The model under review builds one solid part; all positions refer to its coordinate system, in mm. Give positions to 0.01 mm unless a question says otherwise; leave off trailing zeros. Loops run counter-clockwise (first coordinate to the right, second up) from the corner with the lowest first, then second, coordinate; pieces in that order, holes last. Notation, with made-up numbers: (-34.75, -13) - (4.25, -13) arc R29 cw to (4.25, 14) - close; hole circle Ø9 at (48, -36.75). An arc over 180 degrees is marked (long way). Answer as a JSON object with one key per item and string values.
from build123d import *

# Parameters (mm, degrees)
SKETCH1_W           = 12.7
SKETCH1_H           = 12.7
SKETCH1_W_2         = 9.525
SKETCH1_H_2         = 9.525
BOSS_EXTRUDE1_DEPTH = 127
CUT_EXTRUDE1_DEPTH  = 13.7
FILLET1_R           = 1.5875


with BuildPart() as part:
    # Sketch1 → Boss-Extrude1 (new body)
    with BuildSketch(Plane.XY):
        with Locations((6.35, 6.35)):
            Rectangle(SKETCH1_W, SKETCH1_H)
        with Locations((6.35, 6.35)):
            Rectangle(SKETCH1_W_2, SKETCH1_H_2, mode=Mode.SUBTRACT)
    extrude(amount=BOSS_EXTRUDE1_DEPTH)

    # Sketch2 → Cut-Extrude1 (cut, through all)
    with BuildSketch(Plane(origin=(0, 12.7, 0), x_dir=(1, 0, 0), z_dir=(0, 1, 0))):
        Polygon((0, -127), (12.7, -127), (12.7, -114.3), align=None)
    extrude(amount=-CUT_EXTRUDE1_DEPTH, mode=Mode.SUBTRACT)

    # Fillet1
    fillet1_edges = [part.edges().sort_by_distance(p)[0] for p in [
        (12.7, 12.7, 57.15),
        (12.7, 0, 57.15),
        (0, 12.7, 63.5),
        (0, 0, 63.5),
    ]]
    fillet(fillet1_edges, radius=FILLET1_R)


solid = part.part
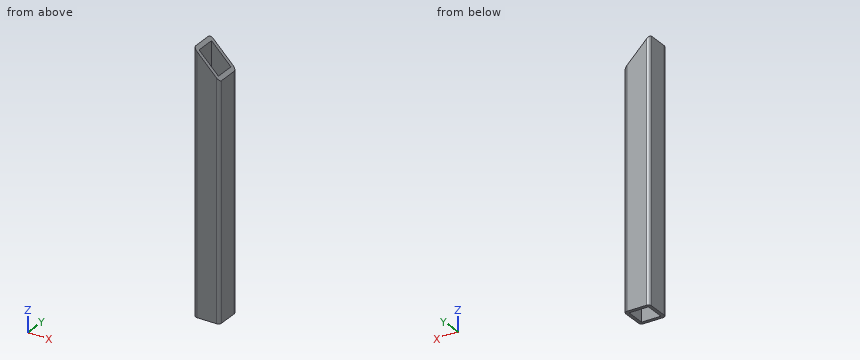
Q1. Consider section B-B, the plane y = 9. State the section outline as (x, z) points, plus the area to 3 significant figures.
Results:
{"outline": "(0, 0) - (1.59, 0) - (1.59, 125.41) - (0, 127) - close; (11.11, 0) - (12.7, 0) - (12.7, 114.3) - (11.11, 115.89) - close", "area": "383 mm^2"}
Q2. Clearance check with a flat-ended pin moving along its axis: pin 1 Ø2 at (x, y) = (1.5, 7.5) entering from +Z. State where the tip first meets the part, or that it passes through.
Results:
{"pin 1": "stops at z = 126.5"}
Q3. Consider section A-A, the plane z = 102.5. State the section outline as (x, y) points (1 decimal).
Results:
{"outline": "(0, 1.6) arc R1.6 ccw to (1.6, 0) - (11.1, 0) arc R1.6 ccw to (12.7, 1.6) - (12.7, 11.1) arc R1.6 ccw to (11.1, 12.7) - (1.6, 12.7) arc R1.6 ccw to (0, 11.1) - close; hole (1.6, 1.6) - (11.1, 1.6) - (11.1, 11.1) - (1.6, 11.1) - close"}
Q4. To check wall thickness, follow probe 1 along X at (y, z) = (11, 68); probe 2 along X at (y, z) = (5, 114.5). State the ranges of each line that lie inside material, in increasing order. Write a range as [from, to].
Results:
{"probe 1": "x = [0, 1.59], [11.11, 12.7]", "probe 2": "x = [0, 1.59], [11.11, 12.5]"}
